Input: part model. Units: mm. Frame: model coordinates. Face numbers are marked on the shaded views. A direction names the side the tool comes from. Coordinates: 2 decimals unless noted, no trailing zeros. Loops run counter-clockwise (first coordinate to the right, second up) from the corner with the lowest first, then second, coordinate; pieces in that order, holes last. Notation, with made-up numbers: (67.5, -20.75) - (122.5, -20.75) arc R36 cw to (122.5, 18.25) - close; hole circle Ø3 at (39.5, 53). An arc over 180 degrees is marked (long way). Use a Markdown table: item, result. Add a question column.
1. Section query A-A on x = 6.5. Return the cut outline in (y, z).
2. Contact query for flat-ended pins moving along their axis: P1, Ø5, axis at y = -16.5, z = 22, coming from the -X side; P2, Ø13, axis at y = 3.5, z = -3.5, coming from the +X side; P3, Ø1.2, axis at y = -0.5, z = -1, coming from the -X side. Output: stop coordinate, or through.
3. Draft query along Z for the marked faces 4, 5 and 6. Return one class per face: released by +Z, released by -Z, zero draft, split by the parting line, or undercut.
4. Ray query, L1, parallel to Y at x = 4.5, z = 0; L2, parallel to Y at x = 15.25, z = 0; L3, parallel to Y at x = 0.5, z = 0. Return the intervals inside material, ascending. Write a range as [from, to].
5. Access query for the marked faces 1, 2 and 3. Directions: +Z, -Z, +X, -X, +Y, -Y. A direction counts if a zero-diameter tool reaches every point of the face in a straight line with its end or side. Return the directions, or none.
6. Section query B-B on y = 0. State how many separate pieces and enclosed holes the cut face has, then the cut area to 3 significant figures.
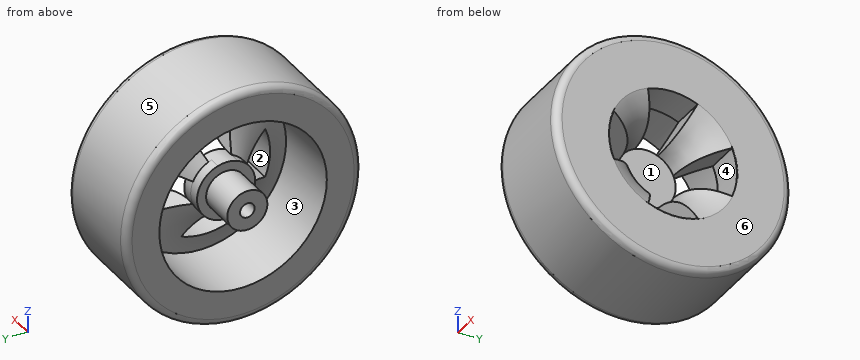
```python
from build123d import *

# Parameters (mm, degrees)
SKETCH_1_R          = 32.5
EXTRUDE_1_DEPTH     = 26.5
SKETCH_2_R          = 23
CUT_EXTRUDE_1_DEPTH = 26.5
CUT_EXTRUDE_START   = -26.5
CUT_EXTRUDE_2_DEPTH = 26.5
FILLET_1_R          = 2


with BuildPart() as part:
    # 草图1 → 凸台-拉伸1 (new body)
    with BuildSketch(Plane(origin=(0, 0, 0), x_dir=(0, 0, -1), z_dir=(1, 0, 0))):
        Circle(SKETCH_1_R)
    extrude(amount=EXTRUDE_1_DEPTH)

    # 草图2 → 切除-拉伸1 (cut)
    with BuildSketch(Plane.ZY):
        Circle(SKETCH_2_R)
    extrude(amount=-CUT_EXTRUDE_1_DEPTH, mode=Mode.SUBTRACT)

    # 草图3 → 旋转2 (revolve)
    with BuildSketch(Plane.XY, mode=Mode.PRIVATE) as revolve_2_sk:
        Polygon((8, 2), (8, 0), (14, 0), (14, 8), (11, 8), (8, 8), (8, 5.5), (-2, 5.5), (-2, 2), align=None)
        with BuildLine():
            Line((11, 8), (14, 8))
            add(Edge.make_bspline(
                [(14, 8), (23.420598, 8.526198), (26.5, 17.699792)],
                knots=[0, 0, 0, 1, 1, 1], degree=2))
            Line((26.5, 17.699792), (26.5, 23))
            Line((26.5, 23), (19.206037, 23))
            add(Edge.make_bspline(
                [(11, 8), (17.176221, 14.336446), (19.206037, 23)],
                knots=[0, 0, 0, 1, 1, 1], degree=2))
        make_face()
    revolve(revolve_2_sk.sketch.rotate(Axis((26.5, 0, 0), (-1, 0, 0)), 270), axis=Axis((26.5, 0, 0), (-1, 0, 0)))

    # 草图4 → 切除-拉伸2 (cut)
    with BuildSketch(Plane(origin=(26.5, 0, 0), x_dir=(0, 0, -1), z_dir=(1, 0, 0)).offset(CUT_EXTRUDE_START)):
        with BuildLine():
            Line((16.230217, -6.759498), (7.377987, -3.092784))
            ThreePointArc((7.377987, -3.092784), (7.999773, 0.060211), (7.330597, 3.20349))
            Line((7.330597, 3.20349), (16.183541, 6.870499))
            ThreePointArc((16.183541, 6.870499), (17.581443, 0.060208), (16.230217, -6.759498))
        make_face()
        with BuildLine():
            Line((-6.759498, -16.230217), (-3.092784, -7.377987))
            ThreePointArc((-3.092784, -7.377987), (0.060211, -7.999773), (3.20349, -7.330597))
            Line((3.20349, -7.330597), (6.870499, -16.183541))
            ThreePointArc((6.870499, -16.183541), (0.060208, -17.581443), (-6.759498, -16.230217))
        make_face()
        with BuildLine():
            Line((-6.870499, 16.183541), (-3.20349, 7.330597))
            ThreePointArc((-3.20349, 7.330597), (-0.060211, 7.999773), (3.092784, 7.377987))
            Line((3.092784, 7.377987), (6.759498, 16.230217))
            ThreePointArc((6.759498, 16.230217), (-0.060208, 17.581443), (-6.870499, 16.183541))
        make_face()
        with BuildLine():
            Line((-16.230217, 6.759498), (-7.377987, 3.092784))
            ThreePointArc((-7.377987, 3.092784), (-7.999773, -0.060211), (-7.330597, -3.20349))
            Line((-7.330597, -3.20349), (-16.183541, -6.870499))
            ThreePointArc((-16.183541, -6.870499), (-17.581443, -0.060208), (-16.230217, 6.759498))
        make_face()
    extrude(amount=CUT_EXTRUDE_2_DEPTH, mode=Mode.SUBTRACT)

    # 圆角1
    fillet_1_edges = [part.edges().sort_by_distance(p)[0] for p in [
        (0, 0, 32.5),
        (26.5, 0, 32.5),
    ]]
    fillet(fillet_1_edges, radius=FILLET_1_R)


solid = part.part
```
Resolved:
| question | item | result |
|---|---|---|
| 1 | outline | circle Ø65 at (0, 0); circle Ø11 at (0, 0); hole circle Ø46 at (0, 0); hole circle Ø4 at (0, 0) |
| 2 | P1 | x = 0 |
| 2 | P2 | x = 22.72 |
| 2 | P3 | x = 8 |
| 3 | face 4 | undercut |
| 3 | face 5 | split by the parting line |
| 3 | face 6 | zero draft |
| 4 | L1 | [-32.5, -23], [-5.5, -2], [2, 5.5], [23, 32.5] |
| 4 | L2 | [-32.5, -23], [23, 32.5] |
| 4 | L3 | [-31.82, -23], [-5.5, -2], [2, 5.5], [23, 31.82] |
| 5 | face 1 | +X |
| 5 | face 2 | +X, -X |
| 5 | face 3 | -X |
| 6 | separate pieces | 3 |
| 6 | enclosed holes | 0 |
| 6 | area | 754 mm² |
